Geometry: see drawing. Coordinates: mm, zero at the bounding-box minimum. A direction names the side the tool comes from. Round coordinates to 2 decimals unless told otherwise and drop trailing zeros. Loops run counter-clockwise (first coordinate to the right, second up) from the corner with the lowest first, then second, coordinate; pieces in that order, holes last. Notation, with made-up numbers: (6, -25) -> (11, -25) arc R15 ccw to (11, -9) -> close; hole circle Ø10 at (86.5, 54). An arc over 180 degrees is marked (long way). Write item = value, one per line.
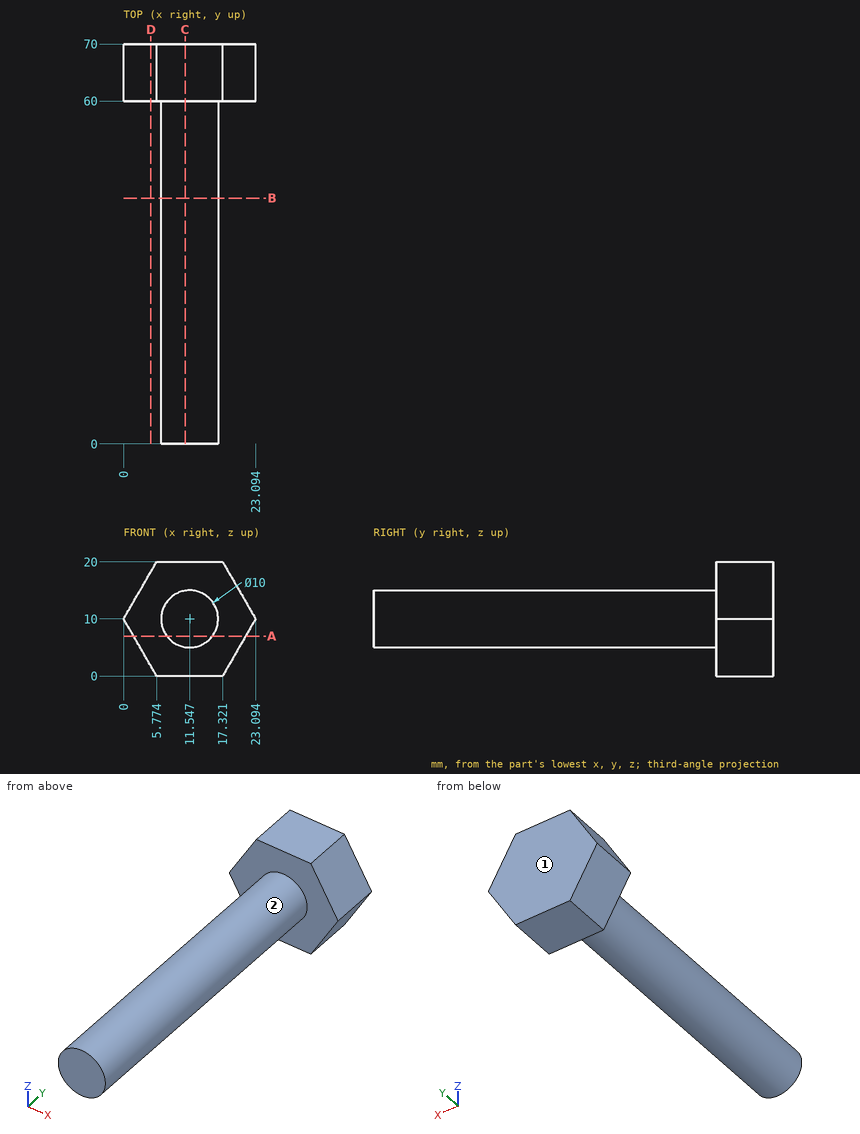
1. Section query C-C (x = 10.75). Return the cut outline in (y, z).
Evaluation:
outline = (0, 5.06) -> (60, 5.06) -> (60, 0) -> (70, 0) -> (70, 20) -> (60, 20) -> (60, 14.94) -> (0, 14.94) -> close
2. Section query B-B (y = 43). Return the cut outline in (x, z).
Evaluation:
outline = circle Ø10 at (11.55, 10)
3. Section query D-D (x = 4.75). Return the cut outline in (y, z).
Evaluation:
outline = (60, 1.77) -> (70, 1.77) -> (70, 18.23) -> (60, 18.23) -> close
4. Line query: probe 1 along Y at (x, z) = (5.5, 1.5); probe 2 along Z at (x, y) = (11.5, 34); probe 3 along Z at (x, y) = (8.75, 19) (1 decimal). Output: solid intervals per line, ascending. Write a range as from..to.
Evaluation:
probe_1 = 60..70
probe_2 = 5..15
probe_3 = 5.9..14.1
5. Contact query for flat-ended pins moving along their axis: pin 1 Ø4 at (x, y) = (15, 36) entering from -Z (1 decimal); pin 2 Ø6 at (x, y) = (10.5, 22) entering from -Z; pin 3 Ø6 at (x, z) = (10.5, 4.5) entering from -Y; pin 4 Ø1.5 at (x, y) = (15, 55.5) entering from +Z (1 decimal). Output: stop coordinate, or through.
Evaluation:
pin_1 = 5.2
pin_2 = 5
pin_3 = 0
pin_4 = 14.2
6. Set-up query: the marked faces 1 and 2. Return all of +Z, -Z, +X, -X, +Y, -Y with unobstructed straight access to the full face (end or side cutting, diameter ignored); none if empty.
Evaluation:
face_1 = +Z, -Z, +X, -X, +Y
face_2 = -Y
7. Section query A-A (z = 7). Return the cut outline in (x, y), then the cut area to 3 significant figures.
Evaluation:
outline = (1.73, 60) -> (7.55, 60) -> (7.55, 0) -> (15.55, 0) -> (15.55, 60) -> (21.36, 60) -> (21.36, 70) -> (1.73, 70) -> close
area = 676 mm²
